The listing builds one solid part. Answer for the finished solid, in the listing's coordinates (mm). A direction names the side the tool comes from. Give positions to 0.01 mm unless a question says otherwise; leave off trailing zeros. Write each loop counter-clockwise with the first axis right and the second up, starting at its lowest first coordinate (ties: lowest second). Pieces come first, ordered by that corner, then holes. Notation, with made-up numbers: (62, 27) -> (110, 27) arc R23 ccw to (110, 50) -> close; hole circle Ø9 at (16.5, 72). An arc over 180 degrees is marked (long way). Put each result on its own line as item: value. Start each with the question number.
1) Find the intervals of material crossed by line 1 along X through (y, z) = (-1, 10.25); line 2 along Y through (x, z) = (23, 5); line 3 along Z through (x, y) = (-14, 11.5), in increasing order. Write a range as from..to.
2) For a pull along Y with two mould halves and no side action, classify faces 1 (the flat face through (-1, -25, 12)), 2 (the flat face through (-1, 0, 2.54)), 3 (the flat face through (-50, 0, 12)) as released by +Y, released by -Y, zero draft, split by the parting line, or undercut.
3) For faces 4 (the flat face through (47.46, 0, 14)), 5 (the flat face through (-4, -24, 25)), determine the directions among +Z, -Z, +X, -X, +Y, -Y from which every point of the face is accessible in a straight line to the end or side of a thin tool.
4) Flat-ended cylindrical pins translate along their axes: pin 1 Ø8 at (x, y) = (11.5, 4) entering from +Z; pin 2 Ø3 at (x, y) = (20, 7) entering from -Z. Find the tip coordinate at first contact, or state that the pin passes through.
5) A cutting plane is placed at A-A (z = 7.5). Write down the section's boundary in (x, y), then the cut area to 3 significant figures.
6) A cutting plane is placed at C-C (y = 21). Write down the section's boundary in (x, z), then the cut area to 3 significant figures.
7) A cutting plane is placed at B-B (x = 32). Write down the section's boundary in (y, z).
from build123d import *

# Parameters (mm, degrees)
F0_W     = 100
F0_H     = 50
F1_DEPTH = 25
F2_T     = -2.54
F3_R     = 7.874883
F4_DEPTH = 25.4


with BuildPart() as f1:
    # F0 (on Top) → F1 (new body)
    with BuildSketch(Plane.XY):
        Rectangle(F0_W, F0_H)
    extrude(amount=F1_DEPTH)

    # F2
    f2_openings = [f1.faces().sort_by_distance(p)[0] for p in [
        (0, 0, 25),
    ]]
    offset(amount=F2_T, openings=f2_openings)

    # F3 (on face) → F4 (cut)
    with BuildSketch(Plane.YZ.offset(50)):
        with Locations((0, 13.071434)):
            Circle(F3_R)
    extrude(amount=F4_DEPTH, mode=Mode.SUBTRACT)


solid = f1.part
Reply:
1. line 1: x = -50..-47.46, 47.46..50
1. line 2: y = -25..-22.46, 22.46..25
1. line 3: z = 0..2.54
2. face 1: released by -Y
2. face 2: undercut
2. face 3: zero draft
3. face 4: +Z
3. face 5: +Z, +X, -X, +Y, -Y
4. pin 1: stops at z = 2.54
4. pin 2: stops at z = 0
5. outline: (-50, -25) -> (50, -25) -> (50, 25) -> (-50, 25) -> close; hole (-47.46, -22.46) -> (47.46, -22.46) -> (47.46, 22.46) -> (-47.46, 22.46) -> close
5. area: 736 mm2
6. outline: (-50, 0) -> (50, 0) -> (50, 25) -> (47.46, 25) -> (47.46, 2.54) -> (-47.46, 2.54) -> (-47.46, 25) -> (-50, 25) -> close
6. area: 368 mm2
7. outline: (-25, 0) -> (25, 0) -> (25, 25) -> (22.46, 25) -> (22.46, 2.54) -> (-22.46, 2.54) -> (-22.46, 25) -> (-25, 25) -> close
